```python
from build123d import *

# Parameters (mm, degrees)
SKETCH1_R           = 11
BOSS_EXTRUDE1_DEPTH = 7
FILLET1_R           = 5


with BuildPart() as part:
    # Sketch1 → Boss-Extrude1 (new body)
    with BuildSketch(Plane.XY):
        with BuildLine():
            Line((-3, 15.716233646), (-3, 81.669056077))
            ThreePointArc((-3, 81.669056077), (0, 81.724137931), (3, 81.669056077))
            Line((3, 81.669056077), (3, 15.716233646))
            ThreePointArc((3, 15.716233646), (13.856406461, 8), (15.110657589, -5.260040611))
            Line((15.110657589, -5.260040611), (72.227477266, -38.236451827))
            ThreePointArc((72.227477266, -38.236451827), (70.775179551, -40.862068966), (69.227477266, -43.43260425))
            Line((69.227477266, -43.43260425), (12.110657589, -10.456193034))
            ThreePointArc((12.110657589, -10.456193034), (0, -16), (-12.110657589, -10.456193034))
            Line((-12.110657589, -10.456193034), (-69.227477266, -43.43260425))
            ThreePointArc((-69.227477266, -43.43260425), (-70.775179551, -40.862068966), (-72.227477266, -38.236451827))
            Line((-72.227477266, -38.236451827), (-15.110657589, -5.260040611))
            ThreePointArc((-15.110657589, -5.260040611), (-13.856406461, 8), (-3, 15.716233646))
        make_face()
        Circle(SKETCH1_R, mode=Mode.SUBTRACT)
    extrude(amount=BOSS_EXTRUDE1_DEPTH)

    # Fillet1
    fillet1_edges = [part.edges().sort_by_distance(p)[0] for p in [
        (-3, 15.716233646, 3.5),
        (3, 15.716233646, 3.5),
        (15.110657589, -5.260040611, 3.5),
        (12.110657589, -10.456193034, 3.5),
        (-12.110657589, -10.456193034, 3.5),
        (-15.110657589, -5.260040611, 3.5),
    ]]
    fillet(fillet1_edges, radius=FILLET1_R)


solid = part.part
```
Geometry: final body of the model. Coordinates: model frame, mm. A direction names the side the tool comes from. Coordinates: 2 decimals unless noted, no trailing zeros. Write each loop counter-clockwise with the first axis right and the second up, starting at its lowest first coordinate (ties: lowest second). Pieces come first, ordered by that corner, then holes. Notation, with made-up numbers: M 36.25,81.5 L 62.25,81.5 A28 cw 62.25,115.5 Z; hole C 75.25,60 d7. An arc over 180 degrees is marked long. Answer as CSV lines item,"result". Start each with the question number.
Q1. Cut plane B-B on y = 0. Return the cut outline in (x, z), then the cut area to 3 significant figures.
Q2. Pin query (flat end, axial travel): P1, Ø1.5, axis at x = -46, z = 4, coming from the -Y side; P2, Ø1, axis at y = 28, z = 3, coming from the +X side; P3, Ø20, axis at x = 0, y = 0, coming from the -Z side; P4, Ø3.5, axis at y = 41.5, z = 3.5, coming from the -X side. Return the tip coordinate at first contact, or that it passes through.
Q3. Cut plane C-C on z = 4.75. Return the cut outline in (x, y), then the cut area to 3 significant figures.
Q4. Line query: line 1 (Y direction, x = 0, z = 3); line 2 (X direction, y = 61.5, z = 5.25); line 3 (X direction, y = -1.5, z = 5). Output: solid intervals per line, ascending. Write a range as from..to.
Q5. Cut plane D-D on y = 70.5. Return the cut outline in (x, z), then the cut area to 3 significant figures.
Q6. Reachability of faces 4 (the flat face through (3, 51, 3)), 5 (the flat face through (42.65, -28.09, 3.45)), 6 (the flat face through (-3, 50, 3)) from +Z, -Z, +X, -X, +Y, -Y: full face, straight path, thin tool, end or side. Return the list, or none.
Q7. Cut plane A-A on x = 0. Return the cut outline in (y, z), then the cut area to 3 significant figures.
Q8. Mould query, pull axis Y, two halves, no side actions, for faces 1 (the flat face through (-41.89, -27.65, 3.45)), 2 (the cylindrical face through (-2.38, -10.74, 3.45)), 3 (the flat face through (-5, 10, 0)). Classes: released by +Y, released by -Y, zero draft, split by the parting line, or undercut.
Findings below:
1,outline,"M -16,0 L -11,0 L -11,7 L -16,7 Z; M 11,0 L 16,0 L 16,7 L 11,7 Z"
1,area,"70.0 mm2"
2,P1,"stops at y = -30.46"
2,P2,"stops at x = 3"
2,P3,"passes through"
2,P4,"stops at x = -3"
3,outline,"M -72.23,-38.24 A81.72 ccw -69.23,-43.43 L -15.32,-12.31 A5 cw -9.76,-12.68 A16 ccw 9.76,-12.68 A5 cw 15.32,-12.31 L 69.23,-43.43 A81.72 ccw 72.23,-38.24 L 18.32,-7.11 A5 cw 15.86,-2.12 A16 ccw 6.1,14.79 A5 cw 3,19.42 L 3,81.67 A81.72 ccw -3,81.67 L -3,19.42 A5 cw -6.1,14.79 A16 ccw -15.86,-2.12 A5 cw -18.32,-7.11 Z; hole C 0,0 d22"
3,area,"1,620 mm2"
4,line 1,"y = -16..-11, 11..81.72"
4,line 2,"x = -3..3"
4,line 3,"x = -15.93..-10.9, 10.9..15.93"
5,outline,"M -3,0 L 3,0 L 3,7 L -3,7 Z"
5,area,"42.0 mm2"
6,face 4,"+Z, -Z, +X, +Y"
6,face 5,"+Z, -Z, -Y"
6,face 6,"+Z, -Z, -X, +Y"
7,outline,"M -16,0 L -11,0 L -11,7 L -16,7 Z; M 11,0 L 81.72,0 L 81.72,7 L 11,7 Z"
7,area,"530 mm2"
8,face 1,"released by -Y"
8,face 2,"undercut"
8,face 3,"zero draft"
